Could you check a few things on this model? Use its own coordinates, in mm. Face numbers are marked on the shaded views. A direction names the side the tool comes from. Give positions to 0.01 mm unless a question says otherwise; leave off trailing zeros. Loops run counter-clockwise (first coordinate to the right, second up) from the corner with the lowest first, then second, coordinate; pieces in that order, holes last. Notation, with made-up numbers: M -37.75,-38.5 L -30.75,-38.5 A24 cw -30.75,-14.5 Z; hole C 26.25,85.25 d3. An arc over 180 degrees is marked long. Use a Markdown table: item, result. Add a question column.
1) Suppose I cut it at B-B on y = -6.5. List the corners of the cut face in (x, z) for me, and give its area (3 significant figures).
2) Will these pins go through, and if not, where does the flat tip stop? pin 1 Ø2.5 at (x, y) = (11.5, 1.5) entering from -Z; pin 2 Ø8 at (x, z) = (-11.5, 0.5) entering from -Y; pin 3 Ø3.5 at (x, z) = (-16, -16.5) entering from -Y.
3) Suppose I cut it at A-A on z = -17. Count the separate pieces of the cut face and the enclosed holes in it, and give its area (3 significant figures).
4) Which directions (+Z, -Z, +X, -X, +Y, -Y) give clear straight access to the entire face, cutting with the end or side of a thin tool? Please do the marked faces 3, 4 and 5.
5) We'd pull the mould along Z, two halves only. Please class the marked faces 1 and 2: +Z half, -Z half, draft (parallel to the pull), parting line (faces both ways), or undercut.
6) Suppose I cut it at D-D on z = 0. List the corners of the cut face in (x, y) for me.
7) If I drill on line 1 along Z through (x, y) = (17, 0.25); line 2 along Z through (x, y) = (17, -0.5); line 3 along X through (y, z) = (-10.5, -4.5), over which ranges is the centre line in solid material (lowest first)? Write a range as [from, to].
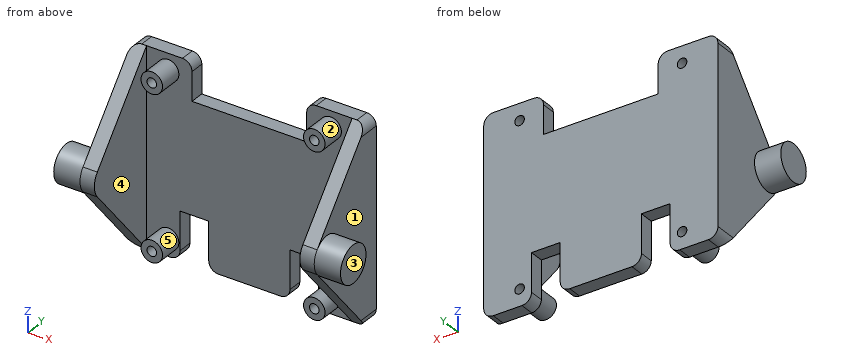
```python
from build123d import *

# Parameters (mm, degrees)
SKETCH_W        = 24.5
SKETCH_H        = 41
PAD_DEPTH       = 3
SKETCH001_R     = 2.25
PAD001_DEPTH    = 5
PAD002_DEPTH    = 3
SKETCH003_R     = 3.9
PAD003_DEPTH    = 5.5
SKETCH004_W     = 12
SKETCH004_H     = 8
POCKET_DEPTH    = 3.001
SKETCH005_W     = 6
SKETCH005_H     = 10
POCKET001_DEPTH = 3.001
SKETCH006_R     = 1
POCKET002_DEPTH = 8.001
FILLET_R        = 2


with BuildPart() as part:
    # Sketch → Pad (new body)
    with BuildSketch(Plane.XZ):
        with Locations((12.25, 0)):
            Rectangle(SKETCH_W, SKETCH_H)
    extrude(amount=-PAD_DEPTH)

    # Sketch001 → Pad001 (join)
    with BuildSketch(Plane.XZ):
        with Locations((17, 17)):
            Circle(SKETCH001_R)
        with Locations((17, -17)):
            Circle(SKETCH001_R)
    extrude(amount=PAD001_DEPTH)

    # Sketch002 (on Face6 of Pad001) → Pad002 (join)
    with BuildSketch(Plane(origin=(24.5, 0, 0), x_dir=(0, 0, 1), z_dir=(1, 0, 0))):
        with BuildLine():
            Line((20.5, 0), (-20.5, 0))
            Line((-20.5, 0), (-2.505853, 15.088428))
            ThreePointArc((2.505853, 15.088428), (0, 16), (-2.505853, 15.088428))
            Line((2.505853, 15.088428), (20.5, 0))
        make_face()
    extrude(amount=-PAD002_DEPTH)

    # Sketch003 (on Face14 of Pad002) → Pad003 (join)
    with BuildSketch(Plane(origin=(24.5, 0, 0), x_dir=(0, 0, 1), z_dir=(1, 0, 0))):
        with Locations((0, 12.1)):
            Circle(SKETCH003_R)
    extrude(amount=PAD003_DEPTH)

    # Sketch004 → Pocket (cut, through all)
    with BuildSketch(Plane.XZ):
        with Locations((6, 16.5)):
            Rectangle(SKETCH004_W, SKETCH004_H)
    extrude(amount=-POCKET_DEPTH, mode=Mode.SUBTRACT)

    # Sketch005 (on Face4 of Pocket) → Pocket001 (cut, through all)
    with BuildSketch(Plane.XZ):
        with Locations((11.5, -15.5)):
            Rectangle(SKETCH005_W, SKETCH005_H)
    extrude(amount=-POCKET001_DEPTH, mode=Mode.SUBTRACT)

    # Sketch006 (on Face20 of Pocket001) → Pocket002 (cut, through all)
    with BuildSketch(Plane.XZ.offset(5)):
        with Locations((17, 17)):
            Circle(SKETCH006_R)
        with Locations((17, -17)):
            Circle(SKETCH006_R)
    extrude(amount=-POCKET002_DEPTH, mode=Mode.SUBTRACT)

    # Fillet
    fillet_edges = [part.edges().sort_by_distance(p)[0] for p in [
        (8.5, 1.5, -20.5),
        (12, 1.5, 20.5),
        (24.5, 1.5, 20.5),
        (24.5, 1.5, -20.5),
        (14.5, 1.5, -20.5),
    ]]
    fillet(fillet_edges, radius=FILLET_R)

    # Mirrored: part across YZ


with BuildPart() as part_1:
    add(part.part)
    add(part.part.mirror(Plane.YZ))


solid = part_1.part
```
Answer block:
| question | item | result |
|---|---|---|
| 1 | outline | M -24.5,-12.75 L -21.5,-12.75 L -21.5,12.75 L -24.5,12.75 Z; M 21.5,-12.75 L 24.5,-12.75 L 24.5,12.75 L 21.5,12.75 Z |
| 1 | area | 153 mm^2 |
| 2 | pin 1 | stops at z = -10.5 |
| 2 | pin 2 | stops at y = 0 |
| 2 | pin 3 | stops at y = -5 |
| 3 | separate pieces | 5 |
| 3 | enclosed holes | 0 |
| 3 | area | 142 mm^2 |
| 4 | face 3 | +Z, -Z, +X, +Y, -Y |
| 4 | face 4 | +Z, -Z, -Y |
| 4 | face 5 | -Y |
| 5 | face 1 | draft |
| 5 | face 2 | undercut |
| 6 | outline | M -30,-16 L -21.5,-16 L -21.5,0 L 21.5,0 L 21.5,-16 L 30,-16 L 30,-8.2 L 24.5,-8.2 L 24.5,3 L -24.5,3 L -24.5,-8.2 L -30,-8.2 Z |
| 7 | line 1 | z = [-20.5, -18], [-16, 16], [18, 20.5] |
| 7 | line 2 | z = [-19.25, -18], [-16, -14.75], [14.75, 16], [18, 19.25] |
| 7 | line 3 | x = [-24.5, -21.5], [21.5, 24.5] |
